Work out the finished part from the listing and answer in its coordinate system (mm). Face numbers are marked on the shaded views. A direction names the side the tool comes from. Coordinates: 2 decimals unless noted, no trailing zeros. Order: outer loops, then holes, each group sorted by start corner. A loop starts at its lowest first (then second) coordinate and runs counter-clockwise, first axis right, second up.
1. Flat-ended cylindrical pins translate along their axes: pin 1 Ø12 at (x, z) = (0, 0) entering from -Y; pin 2 Ø2 at (x, z) = (-10, -7.5) entering from -Y; pin 3 Ø2.5 at (x, z) = (9.9, -9.9) entering from +Y. Find the tip coordinate at first contact, or state that the pin passes through.
2. The part is cut by section A-A, the plane z = 0. Give the vertices of the cut face in (x, y), then the cut area to 3 significant figures.
3. Find the intervals of material crossed by probe 1 along X at (y, z) = (1.5, 10); probe 2 along X at (y, z) = (6, -8); probe 3 along X at (y, z) = (2, -7), in increasing order.
4. The part is cut by section B-B, the plane x = 2. Give the vertices of the cut face in (y, z), then the cut area to 3 significant figures.
5. The part is cut by section C-C, the plane y = 3. Count the separate pieces of the cut face and the enclosed holes in it, then the cut area to 3 significant figures.
6. A tool of negligible diameter and unlimited length cuts with its end or side. For the marked faces 4 and 5, from which of +Z, -Z, +X, -X, +Y, -Y can it reach the whole face along a straight path? Write none if from no direction.
7. Determine the mould class of the marked faces 1, 2 and 3 for opening direction Z: +Z half, -Z half, draft (parallel to the pull), parting line (faces both ways), or undercut.
8. The part is cut by section D-D, the plane y = 6.5. Give the vertices of the cut face in (x, z), then the cut area to 3 significant figures.
```python
from build123d import *

# Parameters (mm, degrees)
SKETCH_1_W               = 32
SKETCH_1_H               = 32
SKETCH_1_R               = 7.5
EXTRUDE_1_DEPTH          = 5
CUT_EXTRUDE_1_DEPTH      = 3.5
SKETCH_3_W               = 32
SKETCH_3_H               = 32
SKETCH_3_W_2             = 30
SKETCH_3_H_2             = 30
EXTRUDE_2_DEPTH          = 2.5
SKETCH_4_R               = 0.85
CUT_EXTRUDE_2_DEPTH      = 8.5
SKETCH_5_R               = 9
CUT_EXTRUDE_3_DEPTH      = 0.5
FILLET_1_R               = 3
SKETCH_6_R               = 0.85
CUT_EXTRUDE_4_DEPTH      = 17
CUT_EXTRUDE_4_DEPTH_BACK = 17
FILLET_2_R               = 1.5


with BuildPart() as part:
    # 草图1 → 凸台-拉伸1 (new body)
    with BuildSketch(Plane(origin=(0, 0, 0), x_dir=(1, 0, 0), z_dir=(0, 1, 0))):
        Rectangle(SKETCH_1_W, SKETCH_1_H)
        with Locations(Location((0, 0, 0), (0, 0, 270))):  # turned: the seam where the file's is
            Circle(SKETCH_1_R, mode=Mode.SUBTRACT)
    extrude(amount=EXTRUDE_1_DEPTH)

    # 草图2 → 切除-拉伸1 (cut)
    with BuildSketch(Plane(origin=(0, 5, 0), x_dir=(1, 0, 0), z_dir=(0, 1, 0))):
        with BuildLine():
            Line((-1.6e-08, 7.5), (-7.5, 7.5))
            Line((-7.5, 7.5), (-7.5, 2.5))
            Line((-7.5, 2.5), (-7.071067812, 2.5))
            ThreePointArc((-7.071067812, 2.5), (-4.330127025, 6.123724352), (-1.6e-08, 7.5))
        make_face()
        with BuildLine():
            Line((7.5, 7.5), (-1.6e-08, 7.5))
            ThreePointArc((-1.6e-08, 7.5), (4.330127013, 6.123724361), (7.071067812, 2.5))
            Line((7.071067812, 2.5), (7.5, 2.5))
            Line((7.5, 2.5), (7.5, 7.5))
        make_face()
        with BuildLine():
            Line((-7.071067812, 2.5), (-7.5, 2.5))
            Line((-7.5, 2.5), (-9, 2.5))
            ThreePointArc((-9, 2.5), (-11.5, 0), (-9, -2.5))
            Line((-9, -2.5), (-7.5, -2.5))
            Line((-7.5, -2.5), (-7.071067812, -2.5))
            ThreePointArc((-7.071067812, -2.5), (-7.5, 0), (-7.071067812, 2.5))
        make_face()
        with BuildLine():
            Line((7.5, 2.5), (7.071067812, 2.5))
            ThreePointArc((7.071067812, 2.5), (7.391989197, 1.26826484), (7.5, 0))
            ThreePointArc((7.5, 0), (7.391989197, -1.26826484), (7.071067812, -2.5))
            Line((7.071067812, -2.5), (7.5, -2.5))
            Line((7.5, -2.5), (9, -2.5))
            ThreePointArc((9, -2.5), (11.5, 0), (9, 2.5))
            Line((9, 2.5), (7.5, 2.5))
        make_face()
        with BuildLine():
            Line((7.5, -2.5), (7.071067812, -2.5))
            ThreePointArc((7.071067812, -2.5), (4.330127019, -6.123724357), (0, -7.5))
            Line((0, -7.5), (7.5, -7.5))
            Line((7.5, -7.5), (7.5, -2.5))
        make_face()
        with BuildLine():
            ThreePointArc((0, -7.5), (-4.330127019, -6.123724357), (-7.071067812, -2.5))
            Line((-7.071067812, -2.5), (-7.5, -2.5))
            Line((-7.5, -2.5), (-7.5, -7.5))
            Line((-7.5, -7.5), (0, -7.5))
        make_face()
    extrude(amount=-CUT_EXTRUDE_1_DEPTH, mode=Mode.SUBTRACT)

    # 草图3 → 凸台-拉伸2 (add)
    with BuildSketch(Plane(origin=(0, 5, 0), x_dir=(1, 0, 0), z_dir=(0, 1, 0))):
        Rectangle(SKETCH_3_W, SKETCH_3_H)
        Rectangle(SKETCH_3_W_2, SKETCH_3_H_2, mode=Mode.SUBTRACT)
    extrude(amount=EXTRUDE_2_DEPTH)

    # 草图4 → 切除-拉伸2 (cut, through all)
    with BuildSketch(Plane.XZ):
        with Locations(Location((-9.899494937, 9.899494937, 0), (0, 0, 270))):  # turned: the seam where the file's is
            Circle(SKETCH_4_R)
        with Locations(Location((9.899494937, 9.899494937, 0), (0, 0, 270))):  # turned: the seam where the file's is
            Circle(SKETCH_4_R)
        with Locations(Location((9.899494937, -9.899494937, 0), (0, 0, 270))):  # turned: the seam where the file's is
            Circle(SKETCH_4_R)
        with Locations(Location((-9.899494937, -9.899494937, 0), (0, 0, 270))):  # turned: the seam where the file's is
            Circle(SKETCH_4_R)
    extrude(amount=-CUT_EXTRUDE_2_DEPTH, mode=Mode.SUBTRACT)

    # 草图5 → 切除-拉伸3 (cut)
    with BuildSketch(Plane.XZ):
        with Locations(Location((0, 0, 0), (0, 0, 270))):  # turned: the seam where the file's is
            Circle(SKETCH_5_R)
    extrude(amount=-CUT_EXTRUDE_3_DEPTH, mode=Mode.SUBTRACT)

    # 圆角1
    fillet_1_edges = [part.edges().sort_by_distance(p)[0] for p in [
        (15, 6.25, -15),
        (-15, 6.25, -15),
        (-15, 6.25, 15),
        (15, 6.25, 15),
        (-16, 3.75, -16),
        (16, 3.75, -16),
        (16, 3.75, 16),
        (-16, 3.75, 16),
    ]]
    fillet(fillet_1_edges, radius=FILLET_1_R)

    # 草图6 → 切除-拉伸4 (cut, two sides)
    with BuildSketch(Plane(origin=(0, 0, 0), x_dir=(0, 0, -1), z_dir=(1, 0, 0))) as cut_extrude_4_sk:
        with Locations((-5.6, 3)):
            Circle(SKETCH_6_R)
        Polygon((-7.656624327, 5), (-3.543375673, 5), (-2.1, 7.5), (-9.1, 7.5), align=None)
    extrude(amount=CUT_EXTRUDE_4_DEPTH, mode=Mode.SUBTRACT)
    extrude(cut_extrude_4_sk.sketch, amount=-CUT_EXTRUDE_4_DEPTH_BACK, mode=Mode.SUBTRACT)

    # 圆角2
    fillet_2_edges = [part.edges().sort_by_distance(p)[0] for p in [
        (-16, 0, 0),
        (0, 0, -16),
        (16, 0, 0),
        (0, 0, 16),
        (-15.121320344, 0, 15.121320344),
        (15.121320344, 0, 15.121320344),
        (15.121320344, 0, -15.121320344),
        (-15.121320344, 0, -15.121320344),
    ]]
    fillet(fillet_2_edges, radius=FILLET_2_R)


solid = part.part
```
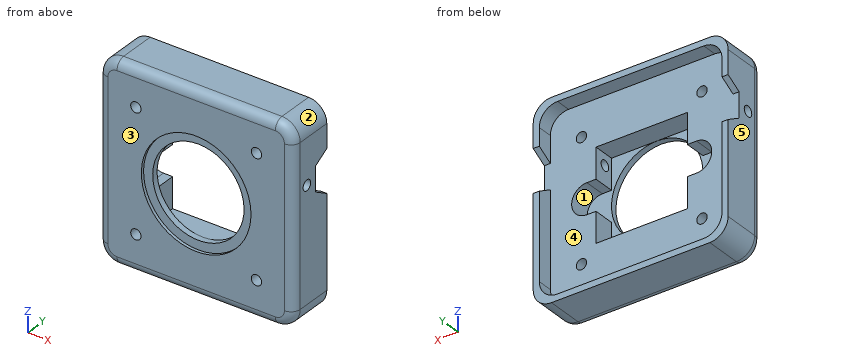
Geometry says:
1. pin 1: passes through
1. pin 2: stops at y = 0
1. pin 3: stops at y = 5
2. outline: (-16, 1.5) arc R1.5 ccw to (-14.5, 0) - (-9, 0) - (-9, 0.5) - (-7.5, 0.5) - (-7.5, 1.5) - (-11.5, 1.5) - (-11.5, 5) - (-15, 5) - (-15, 7.5) - (-16, 7.5) - close; (7.5, 0.5) - (9, 0.5) - (9, 0) - (14.5, 0) arc R1.5 ccw to (16, 1.5) - (16, 7.5) - (15, 7.5) - (15, 5) - (11.5, 5) - (11.5, 1.5) - (7.5, 1.5) - close
2. area: 59.5 mm2
3. probe 1: x = -16 to -10.74, -9.06 to 9.06, 10.74 to 16
3. probe 2: x = -16 to -15, 15 to 16
3. probe 3: x = -16 to -7.5, 7.5 to 16
4. outline: (0, -14.5) arc R1.5 ccw to (1.5, -16) - (7.5, -16) - (7.5, -15) - (5, -15) - (5, -7.5) - (1.5, -7.5) - (1.5, -7.23) - (0.5, -7.23) - (0.5, -8.77) - (0, -8.77) - close; (0, 8.77) - (0.5, 8.77) - (0.5, 7.23) - (1.5, 7.23) - (1.5, 7.5) - (5, 7.5) - (5, 15) - (7.5, 15) - (7.5, 16) - (1.5, 16) arc R1.5 ccw to (0, 14.5) - close
4. area: 88.3 mm2
5. separate pieces: 2
5. enclosed holes: 4
5. area: 719 mm2
6. face 4: +Y
6. face 5: +Z, -Z, -X, +Y, -Y
7. face 1: undercut
7. face 2: +Z half
7. face 3: draft
8. outline: (-16, -13) arc R3 ccw to (-13, -16) - (13, -16) arc R3 ccw to (16, -13) - (16, 2.68) - (15, 2.68) - (15, -12) arc R3 cw to (12, -15) - (-12, -15) arc R3 cw to (-15, -12) - (-15, 2.68) - (-16, 2.68) - close; (-16, 8.52) - (-15, 8.52) - (-15, 12) arc R3 cw to (-12, 15) - (12, 15) arc R3 cw to (15, 12) - (15, 8.52) - (16, 8.52) - (16, 13) arc R3 ccw to (13, 16) - (-13, 16) arc R3 ccw to (-16, 13) - close
8. area: 112 mm2
